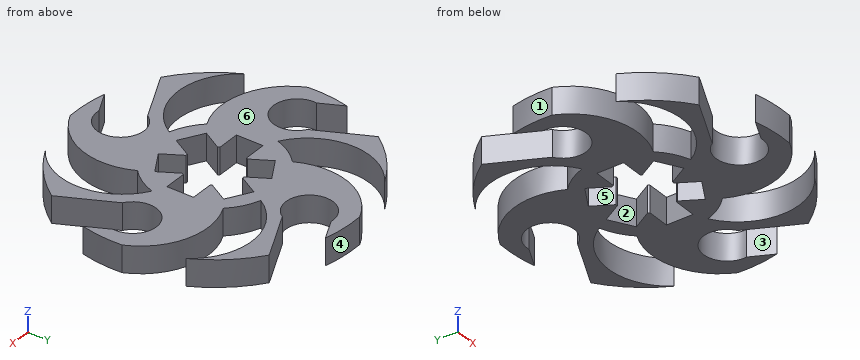
```python
from build123d import *

# Parameters (mm, degrees)
BOSS_EXTRUDE1_DEPTH = 1.524


with BuildPart() as part:
    # Sketch1 → Boss-Extrude1 (new body)
    with BuildSketch(Plane.XY):
        with BuildLine():
            Line((105.591414647, -8.468455362), (106.869091272, -7.853190647))
            ThreePointArc((106.869091272, -7.853190647), (108.22238434, -5.932890961), (105.877274812, -5.793555702))
            Line((105.877274812, -5.793555702), (102.892707432, -7.23077304))
            ThreePointArc((102.892707432, -7.23077304), (101.464153001, -5.925516577), (100.393881735, -4.313380846))
            ThreePointArc((100.393881735, -4.313380846), (103.431247132, -5.892390693), (106.397273409, -4.183136826))
            ThreePointArc((106.397273409, -4.183136826), (105.549139909, -3.783076692), (104.83344904, -3.177135173))
            ThreePointArc((104.83344904, -3.177135173), (101.78471521, -3.345160226), (99.56970685, -1.24355409))
            ThreePointArc((99.56970685, -1.24355409), (99.587627406, -0.043990252), (99.786130504, 1.139171219))
            Line((99.786130504, 1.139171219), (100.401395219, -0.138505406))
            ThreePointArc((100.401395219, -0.138505406), (102.321694905, -1.491798474), (102.461030165, 0.853311054))
            Line((102.461030165, 0.853311054), (101.023812827, 3.837878434))
            ThreePointArc((101.023812827, 3.837878434), (102.32906929, 5.266432866), (103.941205021, 6.336704131))
            ThreePointArc((103.941205021, 6.336704131), (102.362195173, 3.299338734), (104.07144904, 0.333312457))
            ThreePointArc((104.07144904, 0.333312457), (104.471509175, 1.181445957), (105.077450693, 1.897136826))
            ThreePointArc((105.077450693, 1.897136826), (104.90942564, 4.945870656), (107.011031776, 7.160879016))
            ThreePointArc((107.011031776, 7.160879016), (108.210595614, 7.14295846), (109.393757085, 6.944455362))
            Line((109.393757085, 6.944455362), (108.11608046, 6.329190647))
            ThreePointArc((108.11608046, 6.329190647), (106.762787392, 4.408890961), (109.10789692, 4.269555702))
            Line((109.10789692, 4.269555702), (112.092464301, 5.70677304))
            ThreePointArc((112.092464301, 5.70677304), (113.521018732, 4.401516577), (114.591289997, 2.789380846))
            ThreePointArc((114.591289997, 2.789380846), (111.5539246, 4.368390693), (108.587898324, 2.659136826))
            ThreePointArc((108.587898324, 2.659136826), (109.436031823, 2.259076692), (110.151722693, 1.653135173))
            ThreePointArc((110.151722693, 1.653135173), (113.200456523, 1.821160226), (115.415464883, -0.28044591))
            ThreePointArc((115.415464883, -0.28044591), (115.397544326, -1.480009748), (115.199041228, -2.663171219))
            Line((115.199041228, -2.663171219), (114.583776513, -1.385494594))
            ThreePointArc((114.583776513, -1.385494594), (112.663476827, -0.032201526), (112.524141568, -2.377311054))
            Line((112.524141568, -2.377311054), (113.961358906, -5.361878434))
            ThreePointArc((113.961358906, -5.361878434), (112.656102443, -6.790432866), (111.043966712, -7.860704131))
            ThreePointArc((111.043966712, -7.860704131), (112.622976559, -4.823338734), (110.913722693, -1.857312457))
            ThreePointArc((110.913722693, -1.857312457), (110.513662558, -2.705445957), (109.907721039, -3.421136826))
            ThreePointArc((109.907721039, -3.421136826), (110.075746092, -6.469870656), (107.974139956, -8.684879016))
            ThreePointArc((107.974139956, -8.684879016), (106.774576118, -8.66695846), (105.591414647, -8.468455362))
        make_face()
        Polygon((110.207675722, 0), (110.207675722, -1.524), (108.925853356, -1.524), (108.869130969, -1.622246056), (109.510042152, -2.732336789), (108.190219437, -3.494336789), (107.549308253, -2.384246056), (107.435863479, -2.384246056), (106.794952296, -3.494336789), (105.47512958, -2.732336789), (106.116040764, -1.622246056), (106.059318377, -1.524), (104.77749601, -1.524), (104.77749601, 0), (106.059318377, 0), (106.116040764, 0.098246056), (105.47512958, 1.208336789), (106.794952296, 1.970336789), (107.435863479, 0.860246056), (107.549308253, 0.860246056), (108.190219437, 1.970336789), (109.510042152, 1.208336789), (108.869130969, 0.098246056), (108.925853356, 0), align=None, mode=Mode.SUBTRACT)
    extrude(amount=BOSS_EXTRUDE1_DEPTH)


solid = part.part
```
Work out the finished part from the listing and answer in its coordinate system (mm). Face numbers are marked on the shaded views. A direction names the side the tool comes from. Coordinates: 2 decimals unless noted, no trailing zeros. Write each loop counter-clockwise with the first axis right and the second up, starting at its lowest first coordinate (ties: lowest second). Pieces come first, ordered by that corner, then holes.
Q1. Determine the mould class of the marked faces 4, 5 and 6 for opening direction Y: released by +Y, released by -Y, zero draft, split by the parting line, or undercut.
Q2. A cutting plane is placed at B-B, the plane x = 101.75. Give the vertices of the cut face in (y, z), then the cut area to 3 significant figures.
Q3. A cutting plane is placed at A-A, the plane x = 111.5. Give the vertices of the cut face in (y, z), then the cut area to 3 significant figures.
Q4. Which of the six approach directions +Z, -Z, +X, -X, +Y, -Y give full straight-line access (tool end or side, diameter ignored) to the marked faces 1, 2 and 3?
Q5. Find the intervals of material crossed by line 1 (X direction, y = 5.5, z = 1.4); line 2 (Y direction, x = 107, z = 0.85); line 3 (Y direction, x = 105.25, z = 0.2), in increasing order.
Findings below:
1. face 4: released by +Y
1. face 5: undercut
1. face 6: zero draft
2. outline: (-6.24, 0) - (-5.51, 0) - (-5.51, 1.52) - (-6.24, 1.52) - close; (-3.33, 0) - (-1.62, 0) - (-1.62, 1.52) - (-3.33, 1.52) - close; (2.33, 0) - (4.72, 0) - (4.72, 1.52) - (2.33, 1.52) - close
2. area: 7.35 mm2
3. outline: (-7.61, 0) - (-7.5, 0) - (-7.5, 1.52) - (-7.61, 1.52) - close; (-2.3, 0) - (2.04, 0) - (2.04, 1.52) - (-2.3, 1.52) - close; (4.37, 0) - (5.42, 0) - (5.42, 1.52) - (4.37, 1.52) - close
3. area: 8.40 mm2
4. face 1: +Z, -Z, -X
4. face 2: +Z, -Z
4. face 3: +Z, -Z, -Y
5. line 1: x = 102.61 to 103.06, 105.16 to 106.73, 111.66 to 112.37
5. line 2: y = -8.68 to -7.86, -5.17 to -3.14, 1.62 to 4.07, 5.92 to 7.16
5. line 3: y = -6.1 to -5.35, -3.57 to -1.52, 0 to 5.65
